Here's the drawing with two shaded views (mm, measured from the low corner). I have some questions. A direction names the side the tool comes from. Give positions to 0.01 mm unless a question says otherwise; leave off trailing zeros. Loops run counter-clockwise (first coordinate to the right, second up) from the corner with the lowest first, then second, coordinate; pieces in that order, holes last. Notation, with made-up numbers: (20, 81.25) -> (69, 81.25) arc R7 ccw to (69, 86.25) -> close; hole circle Ø11 at (30.5, 82). An arc over 180 degrees is marked (long way). Put each result on its own line as item: value.
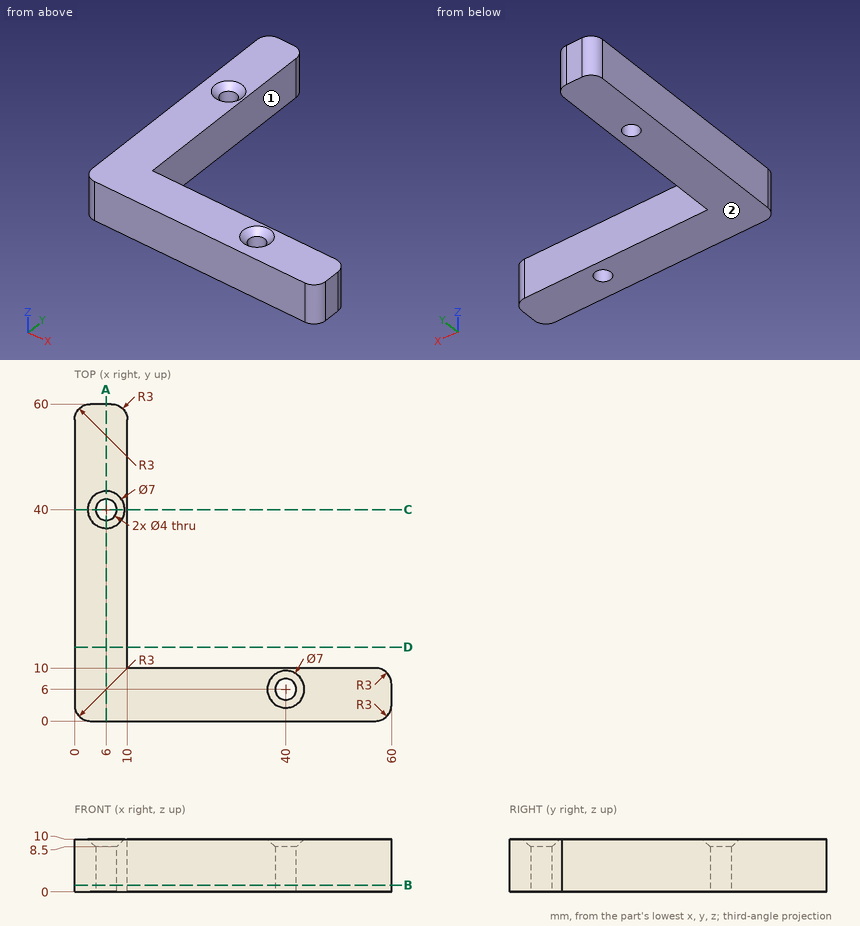
1. For the marked faces 1 and 2, which set-ups out of +Z, -Z, +X, -X, +Y, -Y let a thin tool reach every point of the face, with its end or its side?
Recorded:
face 1: +Z, -Z, +X, +Y
face 2: -Z, +X, -X, +Y, -Y
2. If we section it at A-A (x = 6): List the corners of the cut face in (y, z) for me, then the cut area to 3 significant figures.
Recorded:
outline: (0, 0) -> (38, 0) -> (38, 8.5) -> (36.5, 10) -> (0, 10) -> close; (42, 0) -> (60, 0) -> (60, 10) -> (43.5, 10) -> (42, 8.5) -> close
area: 558 mm^2
3. If we section it at C-C (y = 40): List the corners of the cut face in (x, z) for me, then the cut area to 4 significant figures.
Recorded:
outline: (0, 0) -> (4, 0) -> (4, 8.5) -> (2.5, 10) -> (0, 10) -> close; (8, 0) -> (10, 0) -> (10, 10) -> (9.5, 10) -> (8, 8.5) -> close
area: 57.75 mm^2
4. I'm going to push flat-ended pins straight in: pin 1 (5 mm diameter, centred on x = 42.5, z = 2.5, fed in from +Y); pin 2 (6.5 mm diameter, centred on x = 6, y = 40, fed in from +Z). Where does each tip first touch, or does it pass through?
Recorded:
pin 1: stops at y = 10
pin 2: stops at z = 9.75
5. If we section it at B-B (z = 1.25): List the corners of the cut face in (x, y) for me, then the cut area to 3 significant figures.
Recorded:
outline: (0, 3) arc R3 ccw to (3, 0) -> (57, 0) arc R3 ccw to (60, 3) -> (60, 7) arc R3 ccw to (57, 10) -> (10, 10) -> (10, 57) arc R3 ccw to (7, 60) -> (3, 60) arc R3 ccw to (0, 57) -> close; hole circle Ø4 at (6, 40); hole circle Ø4 at (40, 6)
area: 1,070 mm^2
6. I need wall thicknesses on line 1 (Y direction, x = 6, z = 4); line 2 (Y direction, x = 40, z = 1.5); line 3 (X direction, y = 50, z = 2). Which ranges of each line are inside material? Lowest first, please.
Recorded:
line 1: y = 0 to 38, 42 to 60
line 2: y = 0 to 4, 8 to 10
line 3: x = 0 to 10
7. If we section it at D-D (y = 14): List the corners of the cut face in (x, z) for me, then the cut area to 3 significant figures.
Recorded:
outline: (0, 0) -> (10, 0) -> (10, 10) -> (0, 10) -> close
area: 100 mm^2
